```python
from build123d import *

# Parameters (mm, degrees)
SKETCH1_W                   = 100
SKETCH1_H                   = 38.1
BOSS_EXTRUDE1_DEPTH         = 5
SKETCH2_W                   = 20
SKETCH2_H                   = 12.7
BOSS_EXTRUDE2_DEPTH         = 6
TAP_DRILL_FOR_M4X0_7_TAP1_D = 3.3
SKETCH3_R                   = 2.25
CUT_EXTRUDE1_DEPTH          = 55.625108696
SKETCH12_R                  = 4.5
CUT_EXTRUDE2_DEPTH          = 3
SKETCH13_R                  = 1.75
CUT_EXTRUDE3_DEPTH          = 10


with BuildPart() as part:
    # Sketch1 → Boss-Extrude1 (new body)
    with BuildSketch(Plane(origin=(0, 0, 0), x_dir=(1, 0, 0), z_dir=(0, 1, 0))):
        Rectangle(SKETCH1_W, SKETCH1_H)
    extrude(amount=BOSS_EXTRUDE1_DEPTH)

    # Sketch2 → Boss-Extrude2 (add)
    with BuildSketch(Plane(origin=(0, 5, 0), x_dir=(1, 0, 0), z_dir=(0, 1, 0))):
        with Locations((-26.236645744, 0)):
            Rectangle(SKETCH2_W, SKETCH2_H)
    extrude(amount=BOSS_EXTRUDE2_DEPTH)

    # Tap Drill for M4x0.7 Tap1 (through all)
    with Locations(Plane(origin=(0, 11, 0), x_dir=(1, 0, 0), z_dir=(0, 1, 0))):
        with Locations((-31.236645744, 0), (-21.236645744, 0)):
            Hole(TAP_DRILL_FOR_M4X0_7_TAP1_D / 2)

    # Sketch3 → Cut-Extrude1 (cut, through all)
    with BuildSketch(Plane(origin=(0, 11, 0), x_dir=(1, 0, 0), z_dir=(0, 1, 0))):
        with Locations(Location((-21.236645744, 0, 0), (0, 0, 270))):
            Circle(SKETCH3_R)
        with Locations(Location((-31.236645744, 0, 0), (0, 0, 270))):
            Circle(SKETCH3_R)
    extrude(amount=-CUT_EXTRUDE1_DEPTH, mode=Mode.SUBTRACT)

    # Sketch12 → Cut-Extrude2 (cut)
    with BuildSketch(Plane.XZ):
        with Locations(Location((-31.236645744, 0, 0), (0, 0, 270))):
            Circle(SKETCH12_R)
        with Locations(Location((-21.236645744, 0, 0), (0, 0, 270))):
            Circle(SKETCH12_R)
    extrude(amount=-CUT_EXTRUDE2_DEPTH, mode=Mode.SUBTRACT)

    # Sketch13 → Cut-Extrude3 (cut)
    with BuildSketch(Plane(origin=(0, 5, 0), x_dir=(1, 0, 0), z_dir=(0, 1, 0))):
        with Locations(Location((-46, 15.05, 0), (0, 0, 270))):
            Circle(SKETCH13_R)
        with Locations(Location((-46, -15.05, 0), (0, 0, 270))):
            Circle(SKETCH13_R)
        with Locations(Location((46, -15.05, 0), (0, 0, 270))):
            Circle(SKETCH13_R)
        with Locations(Location((46, 15.05, 0), (0, 0, 270))):
            Circle(SKETCH13_R)
    extrude(amount=-CUT_EXTRUDE3_DEPTH, mode=Mode.SUBTRACT)


solid = part.part
```
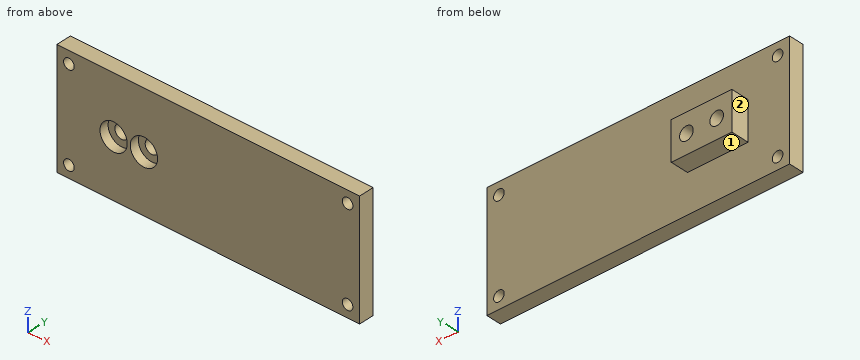
Geometry: final body of the model. Coordinates: model frame, mm. Face numbers are marked on the shaded views. Coordinates: 2 decimals unless noted, no trailing zeros. Order: outer loops, then holes, each group sorted by start corner. A loop starts at its lowest first (then second) coordinate and runs counter-clockwise, first axis right, second up. Notation, with made-up numbers: (33.25, -33) -> (51.25, -33) arc R27 cw to (51.25, -15) -> close; hole circle Ø6 at (26.25, -1). An arc over 180 degrees is marked (long way). Answer in a Markdown table with one row per item.
Item 1: Section D-D on z = -15.05. Output: boundary loops of the cut face in (x, y), plus the area to 3 significant figures.
Return value:
| item | result |
|---|---|
| outline | (-50, 0) -> (-47.75, 0) -> (-47.75, 5) -> (-50, 5) -> close; (-44.25, 0) -> (44.25, 0) -> (44.25, 5) -> (-44.25, 5) -> close; (47.75, 0) -> (50, 0) -> (50, 5) -> (47.75, 5) -> close |
| area | 465 mm² |
Item 2: Ray query, L1, parallel to X at y = 2.7, z = -15.05; L2, parallel to X at y = 4, z = -0.5; L3, parallel to Z at x = -31.5, y = 2.5. Return the intervals inside material, ascending.
Return value:
| item | result |
|---|---|
| L1 | x = -50 to -47.75, -44.25 to 44.25, 47.75 to 50 |
| L2 | x = -50 to -33.43, -29.04 to -23.43, -19.04 to 50 |
| L3 | z = -19.05 to -4.49, 4.49 to 19.05 |
Item 3: Contact query for flat-ended pins moving along their axis: P1, Ø5.5, axis at x = 46, z = 15.05, coming from the -Y side; P2, Ø10, axis at x = -38.5, z = -13.5, coming from the +Y side; P3, Ø3, axis at x = -8.5, y = 7, coming from the +Z side (3 decimals); P4, Ø6.5, axis at x = -23, y = 9.5, coming from the +Z side. Output: stop coordinate, or through.
Return value:
| item | result |
|---|---|
| P1 | stops at y = 0 |
| P2 | stops at y = 5 |
| P3 | passes through |
| P4 | stops at z = 6.35 |
Item 4: Draft query along Z for the marked faces 1 and 2. Return one class per face: released by +Z, released by -Z, zero draft, split by the parting line, or undercut.
Return value:
| item | result |
|---|---|
| face 1 | released by -Z |
| face 2 | zero draft |
Item 5: Section B-B on z = 0. Output: boundary loops of the cut face in (x, y).
Return value:
| item | result |
|---|---|
| outline | (-50, 0) -> (-35.74, 0) -> (-35.74, 3) -> (-33.49, 3) -> (-33.49, 11) -> (-36.24, 11) -> (-36.24, 5) -> (-50, 5) -> close; (-28.99, 3) -> (-26.74, 3) -> (-26.74, 0) -> (-25.74, 0) -> (-25.74, 3) -> (-23.49, 3) -> (-23.49, 11) -> (-28.99, 11) -> close; (-18.99, 3) -> (-16.74, 3) -> (-16.74, 0) -> (50, 0) -> (50, 5) -> (-16.24, 5) -> (-16.24, 11) -> (-18.99, 11) -> close |
Item 6: Section A-A on x = 46. Output: boundary loops of the cut face in (y, z).
Return value:
| item | result |
|---|---|
| outline | (0, -19.05) -> (5, -19.05) -> (5, -16.8) -> (0, -16.8) -> close; (0, -13.3) -> (5, -13.3) -> (5, 13.3) -> (0, 13.3) -> close; (0, 16.8) -> (5, 16.8) -> (5, 19.05) -> (0, 19.05) -> close |
Item 7: Section C-C on y = 2. Output: boundary loops of the cut face in (x, z).
Return value:
| item | result |
|---|---|
| outline | (-50, -19.05) -> (50, -19.05) -> (50, 19.05) -> (-50, 19.05) -> close; hole circle Ø3.5 at (-46, -15.05); hole circle Ø3.5 at (-46, 15.05); hole circle Ø9 at (-31.24, 0); hole circle Ø9 at (-21.24, 0); hole circle Ø3.5 at (46, -15.05); hole circle Ø3.5 at (46, 15.05) |
